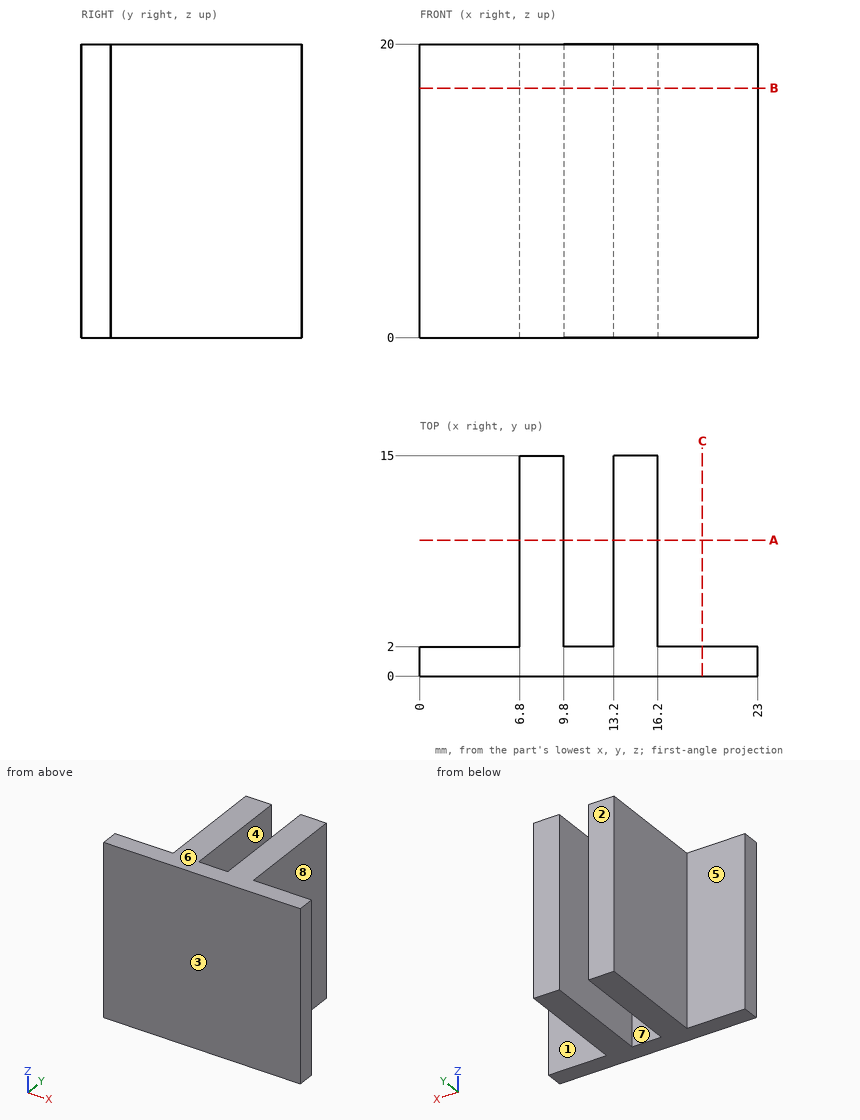
Job drawing, mm, ordinate dimensions from the low corner. One solid piece. A direction names the side the tool comes from. Round coordinates to 2 decimals unless told otherwise and drop trailing zeros. Loops run counter-clockwise (first coordinate to the right, second up) from the corner with the lowest first, then second, coordinate; pieces in that order, holes last. Notation, with made-up numbers: M 15,5 L 43,5 A24 ccw 43,37 Z; hole C -29,43.25 d4. An arc over 180 degrees is marked long. Answer as CSV lines item,"result".
1. 3-axis set-ups, long thin cutter, end or side, ignore diameter. For the marked faces 1, 2, 3, 4 and 5: which of +Z, -Z, +X, -X, +Y, -Y reach the whole face in a straight line?
Resolved:
face 1,"+Z, -Z, +X, +Y"
face 2,"+Z, -Z, +X, -X, +Y"
face 3,"+Z, -Z, +X, -X, -Y"
face 4,"+Z, -Z, +Y"
face 5,"+Z, -Z, -X, +Y"
2. Flat gauge pins, fed straight in: P1, Ø1, axis at x = 12, z = 11, coming from the +Y side; P2, Ø4, axis at y = 10.5, z = 11.5, coming from the +X side. Where does each tip first touch, or does it go through?
Resolved:
P1,"stops at y = 2"
P2,"stops at x = 16.2"
3. Cut at C-C on x = 19.25. Write the cut outline in (y, z), then the cut area to 3 significant figures.
Resolved:
outline,"M 0,0 L 2,0 L 2,20 L 0,20 Z"
area,"40.0 mm²"
4. Cut at A-A on y = 9.25. Write the cut outline in (x, z).
Resolved:
outline,"M 6.8,0 L 9.8,0 L 9.8,20 L 6.8,20 Z; M 13.2,0 L 16.2,0 L 16.2,20 L 13.2,20 Z"
5. Wall check: probe 1 along X at (y, z) = (13.5, 17.25); probe 2 along Y at (x, z) = (20.25, 7). Give the ranges that are in metal, low to high. Write a range as [from, to].
Resolved:
probe 1,"x = [6.8, 9.8], [13.2, 16.2]"
probe 2,"y = [0, 2]"
6. Two-plate mould, pull along X, no slides. Class the marked faces 6, 7 and 8: released by +X, released by -X, zero draft, split by the parting line, or undercut.
Resolved:
face 6,"zero draft"
face 7,"undercut"
face 8,"released by +X"
7. Cut at B-B on z = 17. Write the cut outline in (x, y).
Resolved:
outline,"M 0,0 L 23,0 L 23,2 L 16.2,2 L 16.2,15 L 13.2,15 L 13.2,2 L 9.8,2 L 9.8,15 L 6.8,15 L 6.8,2 L 0,2 Z"
